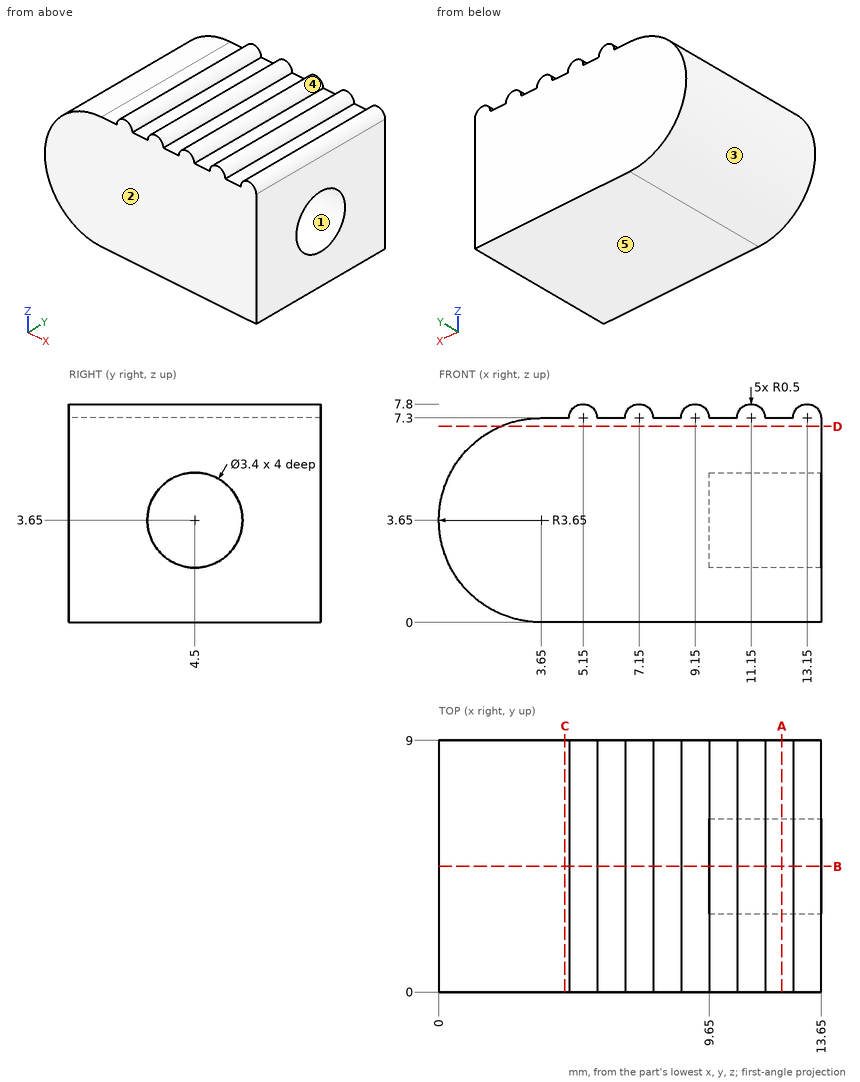
Answer from the drawing. Dimensions are ordinates in mm from the lowest x, y and z of the part. A direction names the side the tool comes from. Coordinates: 2 decimals unless noted, no trailing zeros. Write each loop counter-clockwise with the first axis right and the second up, starting at its lowest first coordinate (ties: lowest second). Pieces come first, ordered by that corner, then holes. Notation, with made-up numbers: (11.25, -11) -> (34.25, -11) arc R21 cw to (34.25, -5) -> close; hole circle Ø6 at (71.5, 14). An arc over 180 degrees is marked (long way). One line per question, with ' | ' between items.
1. Section B-B (y = 4.5) is taken. Determine the outline of the cut face in (x, z), and give its area (3 significant figures).
Verdict:
outline: (3.65, 0) -> (13.65, 0) -> (13.65, 1.95) -> (9.65, 1.95) -> (9.65, 5.35) -> (13.65, 5.35) -> (13.65, 7.3) arc R0.5 ccw to (12.65, 7.3) -> (11.65, 7.3) arc R0.5 ccw to (10.65, 7.3) -> (9.65, 7.3) arc R0.5 ccw to (8.65, 7.3) -> (7.65, 7.3) arc R0.5 ccw to (6.65, 7.3) -> (5.65, 7.3) arc R0.5 ccw to (4.65, 7.3) -> (3.65, 7.3) arc R3.65 ccw to start | area: 82.3 mm^2
2. Section A-A (x = 12.25) is taken. Determine the outline of the cut face in (y, z), and give its area (3 significant figures).
Verdict:
outline: (0, 0) -> (9, 0) -> (9, 7.3) -> (0, 7.3) -> close; hole circle Ø3.4 at (4.5, 3.65) | area: 56.6 mm^2
3. Which of the six approach directions +Z, -Z, +X, -X, +Y, -Y give full straight-line access (tool end or side, diameter ignored) to the marked faces 1 and 2?
Verdict:
face 1: +X | face 2: +Z, -Z, +X, -X, -Y
4. Given pin 1 Ø0.5 at (x, y) = (8, 6.5) entering from +Z; pin 2 Ø1.7 at (y, z) = (4.5, 4) entering from +X, each flat-ended and moving along its own axis, determine where each tip first touches the part or whether it passes through.
Verdict:
pin 1: stops at z = 7.3 | pin 2: stops at x = 9.65
5. Straight lines are drawn through the part: line 1 (Y direction, x = 11.35, z = 3.65); line 2 (Z direction, x = 12.4, y = 4.5); line 3 (X direction, y = 1.5, z = 3.5). For each, find the intervals that lie inside material, in ascending order.
Verdict:
line 1: y = 0 to 2.8, 6.2 to 9 | line 2: z = 0 to 1.95, 5.35 to 7.3 | line 3: x = 0 to 13.65
6. Section C-C (x = 4.5) is taken. Determine the outline of the cut face in (y, z), and give its area (3 significant figures).
Verdict:
outline: (0, 0) -> (9, 0) -> (9, 7.3) -> (0, 7.3) -> close | area: 65.7 mm^2
7. For a pull along X with two mould halves and no side action, classify the marked faces 3, 4 and 5 as released by +X, released by -X, zero draft, split by the parting line, or undercut.
Verdict:
face 3: released by -X | face 4: undercut | face 5: zero draft
8. Section D-D (z = 7) is taken. Determine the outline of the cut face in (x, y), and give its area (3 significant figures).
Verdict:
outline: (2.2, 0) -> (13.65, 0) -> (13.65, 9) -> (2.2, 9) -> close | area: 103 mm^2
